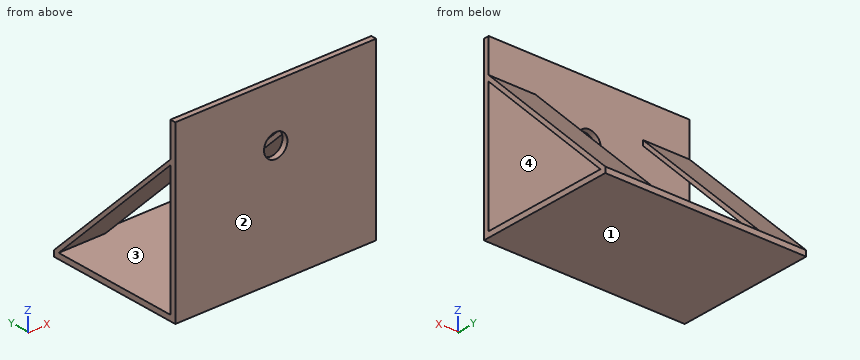
from build123d import *

# Parameters (mm, degrees)
F0_W     = 54.61
F0_H     = 38.1
F1_DEPTH = 1.524
F2_W     = 54.61
F2_H     = 1.524
F3_DEPTH = 45.72
F4_R     = 3.175
F5_DEPTH = 25.4
F7_DEPTH = 12.7
F9_DEPTH = 12.7


with BuildPart() as f1:
    # F0 (on Top) → F1 (new body)
    with BuildSketch(Plane.XY):
        Rectangle(F0_W, F0_H)
    extrude(amount=F1_DEPTH)

    # F2 (on face) → F3 (join)
    with BuildSketch(Plane.XY.offset(1.524)):
        with Locations((0, -18.288)):
            Rectangle(F2_W, F2_H)
    extrude(amount=F3_DEPTH)

    # F4 (on face) → F5 (cut)
    with BuildSketch(Plane.XZ.offset(19.05)):
        with Locations((0, 32.004)):
            Circle(F4_R)
    extrude(amount=-F5_DEPTH, mode=Mode.SUBTRACT)

    # F6 (on face) → F7 (join)
    with BuildSketch(Plane.YZ.offset(27.305)):
        Polygon((17.526, 1.524), (19.05, 1.524), (-17.526, 38.1), (-17.526, 36.576), align=None)
    extrude(amount=-F7_DEPTH)

    # F8 (on face) → F9 (join)
    with BuildSketch(Plane(origin=(-27.305, 0, 0), x_dir=(0, -1, 0), z_dir=(-1, 0, 0))):
        Polygon((17.526, 37.915688), (-19.05, 1.524), (-17.526, 1.524), (17.526, 36.576), align=None)
    extrude(amount=-F9_DEPTH)


solid = f1.part
The listing builds one solid part. Answer for the finished solid, in the listing's coordinates (mm). Face numbers are marked on the shaded views. Give positions to 0.01 mm unless a question says otherwise; leave off trailing zeros. Loops run counter-clockwise (first coordinate to the right, second up) from the corner with the lowest first, then second, coordinate; pieces in that order, holes last. Notation, with made-up numbers: (61.25, 74) - (68.25, 74) arc R25 ccw to (68.25, 87) - close; hole circle Ø9 at (85.25, 10). An arc over 180 degrees is marked (long way). Use one line per item in the form item = value.
1. Section B-B on y = 12 is taken. Give the vertices of the cut face in (x, z) (3 decimals), then the cut area to 3 significant figures.
Calculated:
outline = (-27.305, 0) - (27.305, 0) - (27.305, 1.524) - (-27.305, 1.524) - close; (-27.305, 7.05) - (-14.605, 7.05) - (-14.605, 8.538) - (-27.305, 8.538) - close; (14.605, 7.05) - (27.305, 7.05) - (27.305, 8.574) - (14.605, 8.574) - close
area = 121 mm^2
2. Section D-D on x = 0 is taken. Give the vertices of the cut face in (y, z).
Calculated:
outline = (-19.05, 0) - (19.05, 0) - (19.05, 1.52) - (-17.53, 1.52) - (-17.53, 28.83) - (-19.05, 28.83) - close; (-19.05, 35.18) - (-17.53, 35.18) - (-17.53, 47.24) - (-19.05, 47.24) - close
3. The mould has two halves that part along Y. Classify the marked faces 1, 2, 3 and 4: pulls with the +Y half, pulls with the -Y half, needs draft (parallel to the pull), parting line crosses it, or undercut.
Calculated:
face_1 = needs draft
face_2 = pulls with the -Y half
face_3 = undercut
face_4 = undercut
4. Section A-A on x = 15.5 is taken. Give the vertices of the cut face in (y, z).
Calculated:
outline = (-19.05, 0) - (19.05, 0) - (19.05, 1.52) - (-17.53, 38.1) - (-17.53, 47.24) - (-19.05, 47.24) - close; hole (-17.53, 1.52) - (17.53, 1.52) - (-17.53, 36.58) - close
5. Find the intervals of material crossed by line 1 along X through (y, z) = (-6.5, 26) (3 decimals); line 2 along Z through (x, y) = (0, -18.4); line 3 along Y through (x, z) = (6, 36.5), in increasing order. Write a range as [from, to].
Calculated:
line_1 = [-27.305, -14.605], [14.605, 27.305]
line_2 = [0, 28.83], [35.18, 47.24]
line_3 = [-19.05, -17.53]
6. Given pin 1 Ø12 at (x, y) = (-5, -13) entering from -Z; pin 2 Ø23 at (x, z) = (-1, 17.5) entering from +Y; pin 3 Ø8 at (x, y) = (9.5, 7.5) entering from +Z; pin 4 Ø11 at (x, y) = (-12.5, 9.5) entering from +Z, each flat-ended and moving along its own axis, determine where each tip first touches the part or whether it passes through.
Calculated:
pin_1 = 0
pin_2 = -17.53
pin_3 = 1.52
pin_4 = 16.08
7. Section C-C on z = 8 is taken. Give the vertices of the cut face in (x, y) (3 decimals), then the cut area to 3 significant figures.
Calculated:
outline = (-27.305, -19.05) - (27.305, -19.05) - (27.305, -17.526) - (-27.305, -17.526) - close; (-27.305, 11.05) - (-14.605, 11.05) - (-14.605, 12.541) - (-27.305, 12.541) - close; (14.605, 11.05) - (27.305, 11.05) - (27.305, 12.574) - (14.605, 12.574) - close
area = 122 mm^2
